```python
from build123d import *

# Parameters (mm, degrees)
BOSS_EXTRUDE1_DEPTH = 27.94
SKETCH2_W           = 5.576427518
SKETCH2_H           = 7.825401813
BOSS_EXTRUDE4_DEPTH = 29.21
SKETCH8_W           = 10.146325875
SKETCH8_H           = 25.699088163
CUT_EXTRUDE2_DEPTH  = 7.606325874
SKETCH10_W          = 4.931914879
SKETCH10_H          = 2.216881434
CUT_EXTRUDE3_DEPTH  = 7.606325874


with BuildPart() as part:
    # 3DSketch1 → Boss-Extrude1 (new body)
    with BuildSketch(Plane(origin=(-4.102739017, 20.36405405, 0.057228779), x_dir=(0.8412817346270438, -0.540596932087958, 0), z_dir=(0, 0, -1))):
        Polygon((0, 0), (4.230388213, 6.583367612), (14.475483209, 0), (10.245094996, -6.583367612), align=None)
    extrude(amount=-BOSS_EXTRUDE1_DEPTH)

    # Sketch2 → Boss-Extrude4 (add)
    with BuildSketch(Plane.XY):
        with Locations((1.905853526, 16.451353144)):
            Rectangle(SKETCH2_W, SKETCH2_H)
    extrude(amount=BOSS_EXTRUDE4_DEPTH)

    # Sketch8 → Cut-Extrude2 (cut)
    with BuildSketch(Plane(origin=(0, 20.36405405, 0), x_dir=(1, 0, 0), z_dir=(0, 1, 0))):
        with Locations((2.022741779, -13.698787424)):
            Rectangle(SKETCH8_W, SKETCH8_H)
    extrude(amount=-CUT_EXTRUDE2_DEPTH, mode=Mode.SUBTRACT)

    # Sketch10 → Cut-Extrude3 (cut)
    with BuildSketch(Plane(origin=(0, 20.36405405, 0), x_dir=(1, 0, 0), z_dir=(0, 1, 0))):
        with Locations((1.837563479, -27.656772222)):
            Rectangle(SKETCH10_W, SKETCH10_H)
    extrude(amount=-CUT_EXTRUDE3_DEPTH, mode=Mode.SUBTRACT)


solid = part.part
```
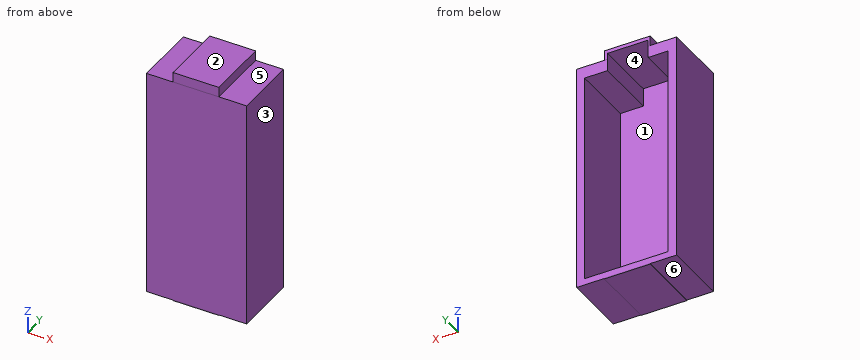
CAD build for the part. Positions are in the model's coordinates, mm. Face numbers are marked on the shaded views. A direction names the side the tool comes from. Round coordinates to 2 decimals unless told otherwise and drop trailing zeros. Order: outer loops, then holes, each group sorted by start corner. A loop starts at its lowest first (then second) coordinate and runs counter-clockwise, first axis right, second up. Notation, with made-up numbers: (34, 20) - (47, 20) arc R29 ccw to (47, 52) - close; hole circle Ø8 at (50.5, 9.25). An arc over 180 degrees is marked (long way). Answer in a Markdown table with one row per item. Add a question column.
(1) 3-axis set-ups, long thin cutter, end or side, ignore diameter. For the marked faces 4, 5 and 6: which of +Z, -Z, +X, -X, +Y, -Y reach the whole face in a straight line?
(2) Drop flat-ended pins along their axis: pin 1 Ø3 at (x, y) = (0.5, 16) entering from -Z; pin 2 Ø5 at (x, z) = (-0.5, 14.5) entering from +Y; pin 3 Ø1.7 at (x, y) = (7, 15.5) entering from +Z; pin 4 Ø1.4 at (x, y) = (5.5, 18) entering from -Z. Give the stop position or say it passes through.
(3) Band-saw the part on C-C on z = 7.5. List the corners of the cut face in (x, y), and give its area (3 significant figures).
(4) Band-saw the part on A-A on y = 16.75. List the corners of the cut face in (x, z), and give its area (3 significant figures).
(5) Band-saw the part on B-B on x = 4. List the corners of the cut face in (y, z).
(6) Band-saw the part on D-D on x = 5.75. List the corners of the cut face in (y, z).
(7) Mould opens along X. For the marked faces 1, 2 and 3 say: +X half, -X half, draft (parallel to the pull), parting line (faces both ways), or undercut.
(8) Probe L1, parallel to X at y = 15, z = 17.75; L2, parallel to Z at x = 3.25, y = 19.5; L3, parallel to X at y = 15.5, z = 27. List the from-to ranges inside material, lowest first. Write a range as [from, to].
Data:
| question | item | result |
|---|---|---|
| 1 | face 4 | +Y |
| 1 | face 5 | +Z, +X, +Y, -Y |
| 1 | face 6 | -Z, -X, +Y, -Y |
| 2 | pin 1 | stops at z = 0 |
| 2 | pin 2 | stops at y = 12.76 |
| 2 | pin 3 | stops at z = 28 |
| 2 | pin 4 | stops at z = 0.06 |
| 3 | outline | (-4.1, 12.54) - (8.08, 12.54) - (8.08, 20.36) - (7.1, 20.36) - (7.1, 12.76) - (-3.05, 12.76) - (-3.05, 20.36) - (-4.1, 20.36) - close |
| 3 | area | 18.1 mm^2 |
| 4 | outline | (-4.1, 0.06) - (-0.88, 0.06) - (-0.88, 0) - (4.69, 0) - (4.69, 0.06) - (8.08, 0.06) - (8.08, 28) - (4.69, 28) - (4.69, 29.21) - (-0.88, 29.21) - (-0.88, 28) - (-4.1, 28) - close; hole (-3.05, 0.85) - (7.1, 0.85) - (7.1, 26.55) - (4.3, 26.55) - (4.3, 28.77) - (-0.63, 28.77) - (-0.63, 26.55) - (-3.05, 26.55) - close |
| 4 | area | 75.6 mm^2 |
| 5 | outline | (12.54, 0) - (20.36, 0) - (20.36, 0.85) - (12.76, 0.85) - (12.76, 28.77) - (20.36, 28.77) - (20.36, 29.21) - (12.54, 29.21) - close |
| 6 | outline | (12.54, 0.06) - (20.36, 0.06) - (20.36, 0.85) - (12.76, 0.85) - (12.76, 26.55) - (20.36, 26.55) - (20.36, 28) - (12.54, 28) - close |
| 7 | face 1 | undercut |
| 7 | face 2 | draft |
| 7 | face 3 | +X half |
| 8 | L1 | x = [-4.1, -3.05], [7.1, 8.08] |
| 8 | L2 | z = [0, 0.85], [28.77, 29.21] |
| 8 | L3 | x = [-4.1, -0.63], [4.3, 8.08] |
